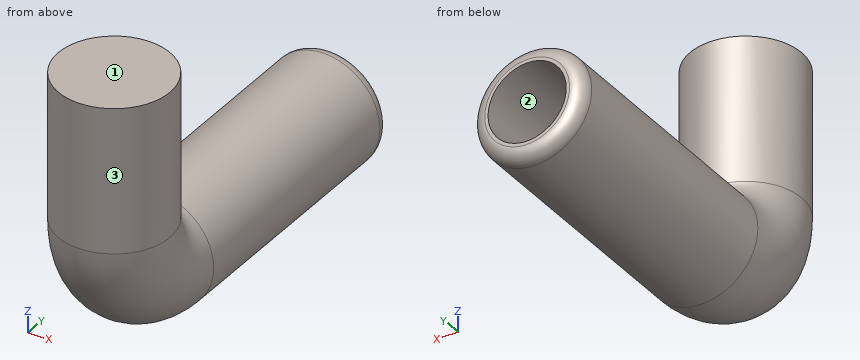
```python
from build123d import *

# Parameters (mm, degrees)
SWEEP1_PROFILE_R    = 25
BOSS_EXTRUDE2_START = 30
SKETCH32_R          = 25
SKETCH32_R_2        = 17.5
BOSS_EXTRUDE2_DEPTH = 30
FILLET1_R           = 6
SKETCH33_R          = 17.5
CUT_EXTRUDE1_DEPTH  = 80


with BuildPart() as part:
    # Sweep1: sweep along a path in Sketch2
    with BuildLine(Plane(origin=(0, 0, 0), x_dir=(0, 0, -1), z_dir=(1, 0, 0))) as sweep1_path:
        Line((-65, 0), (0, 0))
        ThreePointArc((0, 0), (21.213203436, 8.786796564), (30, 30))
        Line((30, 30), (30, 120))
    # Sweep1 profile (on start of the path) → Sweep1 (sweep)
    with BuildSketch(Plane(origin=(0, 0, 65), x_dir=(-1, 0, 0), z_dir=(0, 0, -1))):
        Circle(SWEEP1_PROFILE_R)
    sweep(path=sweep1_path.line)

    # Sketch32 → Boss-Extrude2 (add)
    with BuildSketch(Plane(origin=(0, 120, 0), x_dir=(1, 0, 0), z_dir=(0, 1, 0)).offset(BOSS_EXTRUDE2_START)):
        with Locations(Location((0, 30, 0), (0, 0, 270))):
            Circle(SKETCH32_R)
        with Locations(Location((0, 30, 0), (0, 0, 270))):
            Circle(SKETCH32_R_2, mode=Mode.SUBTRACT)
    extrude(amount=-BOSS_EXTRUDE2_DEPTH)

    # Fillet1
    fillet1_edges = [part.edges().sort_by_distance(p)[0] for p in [
        (0, 150, -55),
    ]]
    fillet(fillet1_edges, radius=FILLET1_R)

    # Sketch33 → Cut-Extrude1 (cut)
    with BuildSketch(Plane(origin=(0, 120, 0), x_dir=(1, 0, 0), z_dir=(0, 1, 0))):
        with Locations(Location((0, 30, 0), (0, 0, 270))):
            Circle(SKETCH33_R)
    extrude(amount=-CUT_EXTRUDE1_DEPTH, mode=Mode.SUBTRACT)


solid = part.part
```
Model file for the job. Use its own axes, mm. Face numbers are marked on the shaded views. A direction names the side the tool comes from. Coordinates: 2 decimals unless noted, no trailing zeros. Order: outer loops, then holes, each group sorted by start corner. A loop starts at its lowest first (then second) coordinate and runs counter-clockwise, first axis right, second up. Notation, with made-up numbers: (-5.75, -40) -> (44.25, -40) arc R19 ccw to (44.25, -25) -> close; hole circle Ø10 at (89.5, 84). An arc over 180 degrees is marked (long way). Answer as a JSON object with one key per item and string values. Group by question number.
1) Flat gauge pins, fed straight in: pin 1 (10 mm diameter, centred on x = -16, y = 117, fed in from -Z); pin 2 (2 mm diameter, centred on x = -5, z = -15, fed in from -Y); pin 3 (2 mm diameter, centred on x = -1.5, y = 66.5, fed in from +Z) (3 decimals). Where does each tip first touch, or does it go through?
2) Cut at B-B, the plane z = 22. Write the cut outline in (x, y), then the cut area to 3 significant figures.
3) Cut at A-A, the plane y = 45. Write the cut outline in (x, z), then the cut area to 3 significant figures.
4) Which spindle directions (+Z, -Z, +X, -X, +Y, -Y) get a long thin tool onto all of the face, cutting with end or side? Do the marked faces 1, 2 and 3. Say none if no direction does.
5) Drill centre lines: L1, parallel to X at y = 88, z = -30; L2, parallel to Z at x = 9, y = 118; L3, parallel to Y at x = -1, z = 7. Where is each one in solid material? Low to high.
Check values:
{
 "1": {"pin 1": "stops at z = -52.45", "pin 2": "stops at y = -22.73", "pin 3": "stops at z = -5.005"},
 "2": {"outline": "circle Ø50 at (0, 0)", "area": "1,960 mm²"},
 "3": {"outline": "circle Ø50 at (0, -30); hole circle Ø35 at (0, -30)", "area": "1,000 mm²"},
 "4": {"face 1": "+Z, +X, -X, +Y, -Y", "face 2": "+Y", "face 3": "+Z"},
 "5": {"L1": "x = -25 to -17.5, 17.5 to 25", "L2": "z = -53.32 to -45.01, -14.99 to -6.68", "L3": "y = -24.98 to 24.98"}
}
